from build123d import *

# Parameters (mm, degrees)
F0_W     = 50
F0_H     = 20
F1_DEPTH = 100
F2_SIZE2 = 39.99999
F2_SIZE  = 19.99999
F3_W     = 40
F3_H     = 20
F4_DEPTH = 20
F5_W     = 40
F5_H     = 20
F6_DEPTH = 20


# Not quite as in the source:
# - a fillet or chamfer is up to 0.001 mm smaller than in the source, because OpenCascade refuses the exact size


with BuildPart() as f1:
    # F0 (on Front) → F1 (new body)
    with BuildSketch(Plane.XZ):
        Rectangle(F0_W, F0_H)
    extrude(amount=F1_DEPTH)

    # F2 (size 20 and 40 in the source; OpenCascade refuses exactly that, so slightly less here)
    f2_edges = [f1.edges().sort_by_distance(p)[0] for p in [
        (0, -100, 10),
    ]]
    f2_side = f1.faces().sort_by_distance((0, -100, 0))[0]
    chamfer(f2_edges, length=F2_SIZE, length2=F2_SIZE2, reference=f2_side)

    # F3 (on face) → F4 (join)
    with BuildSketch(Plane.YZ.offset(25)):
        with Locations((-20, 0)):
            Rectangle(F3_W, F3_H)
    extrude(amount=F4_DEPTH)

    # F5 (on face) → F6 (join)
    with BuildSketch(Plane(origin=(-25, 0, 0), x_dir=(0, -1, 0), z_dir=(-1, 0, 0))):
        with Locations((20, 0)):
            Rectangle(F5_W, F5_H)
    extrude(amount=F6_DEPTH)


solid = f1.part
For this review, take the finished solid that the model builds, in its own axes (mm). A direction names the side the tool comes from. Give positions to 0.01 mm unless a question says otherwise; leave off trailing zeros. Order: outer loops, then holes, each group sorted by start corner. A loop starts at its lowest first (then second) coordinate and runs counter-clockwise, first axis right, second up. Notation, with made-up numbers: (63.25, 69.25) -> (117.25, 69.25) arc R28 ccw to (117.25, 95.25) -> close; hole circle Ø3 at (-7, 33). An arc over 180 degrees is marked (long way). Write item = value, one per line.
1) Insertion check: pin 1 (6 mm diameter, centred on x = -3.5, z = 0.5, fed in from -Y); pin 2 (3 mm diameter, centred on x = -10, z = 5.5, fed in from -Y). Each pin has a flat end and moves straight along its axis. Give the tip position at first contact, or say it passes through.
Findings:
pin_1 = -85
pin_2 = -72
2) We need section C-C, the plane y = -80.5. Give the boundary of the cut face in (x, z), and give its area (4 significant figures).
Findings:
outline = (-25, -10) -> (25, -10) -> (25, -0.25) -> (-25, -0.25) -> close
area = 487.5 mm^2
3) For faces 4 (the face through (-35, -40, 0)), 5 (the face through (25, -63, -2)), 6 (the face through (1, -38, -10)), list the 3-axis set-ups (+Z, -Z, +X, -X, +Y, -Y) from which the entire face can be reached by the end or side of a thin tool; tool diameter is ignored.
Findings:
face_4 = +Z, -Z, -X, -Y
face_5 = +Z, -Z, +X, -Y
face_6 = -Z, +X, -X, +Y, -Y
4) Draft analysis for pull direction Y (two halves, no side actions). For faces 1 (the face through (1, 0, 0)), 2 (the face through (-45, -20, 0)), 3 (the face through (35, -40, 0)), state which applies: pulls with the +Y half, pulls with the -Y half, needs draft (parallel to the pull), parting line crosses it, or undercut.
Findings:
face_1 = pulls with the +Y half
face_2 = needs draft
face_3 = pulls with the -Y half
5) We need section A-A, the plane z = 3. Give the boundary of the cut face in (x, y).
Findings:
outline = (-45, -40) -> (-25, -40) -> (-25, -74) -> (25, -74) -> (25, -40) -> (45, -40) -> (45, 0) -> (-45, 0) -> close
6) To check wall thickness, follow L1, parallel to X at y = -63, z = 6.75; L2, parallel to Y at x = 40.5, z = 8.5; L3, parallel to Y at x = 10, z = -0.5. State the ranges of each line that lie inside material, in increasing order. Write a range as from..to.
Findings:
L1 = -25..25
L2 = -40..0
L3 = -81..0
7) We need section D-D, the plane z = -7.75. Give the boundary of the cut face in (x, y).
Findings:
outline = (-45, -40) -> (-25, -40) -> (-25, -95.5) -> (25, -95.5) -> (25, -40) -> (45, -40) -> (45, 0) -> (-45, 0) -> close
